Could you check a few things on this drawing? It's one solid part, dimensions in mm from its lowest x, y, z. Give positions to 0.01 mm unless a question says otherwise; leave off trailing zeros. Loops run counter-clockwise (first coordinate to the right, second up) from the corner with the lowest first, then second, coordinate; pieces in that order, holes last. Notation, with made-up numbers: (-23.5, -39.75) - (25.5, -39.75) arc R21 ccw to (25.5, -29.75) - close; hole circle Ø4 at (19, 67). An arc over 180 degrees is marked (long way). Use a Markdown table: item, result.
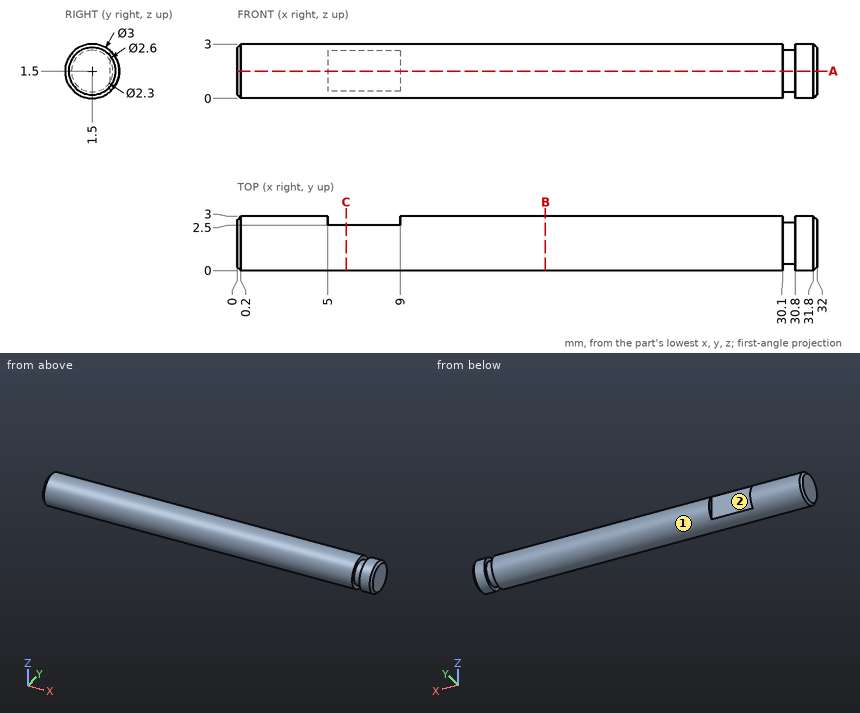
(1) Will this pin go through, and if not, where does the flat tip stop? pin 1 (0.7 mm diameter, centred on x = 6.5, z = 1.5, fed in from +Y).
A:
| item | result |
|---|---|
| pin 1 | y = 2.5 |
(2) Suppose I cut it at C-C on x = 6. Write out the boundary of the cut face in (y, z).
A:
| item | result |
|---|---|
| outline | (2.5, 0.38) - (2.5, 2.62) arc R1.5 ccw (long way) to start |
(3) Suppose I cut it at A-A on z = 1.5. Write out the boundary of the cut face in (x, y), plus the area to 3 significant figures.
A:
| item | result |
|---|---|
| outline | (0, 0.2) - (0.2, 0) - (30.1, 0) - (30.1, 0.35) - (30.8, 0.35) - (30.8, 0) - (31.8, 0) - (32, 0.2) - (32, 2.8) - (31.8, 3) - (30.8, 3) - (30.8, 2.65) - (30.1, 2.65) - (30.1, 3) - (9, 3) - (9, 2.5) - (5, 2.5) - (5, 3) - (0.2, 3) - (0, 2.8) - close |
| area | 93.4 mm2 |
(4) Suppose I cut it at B-B on x = 17. Write out the boundary of the cut face in (y, z).
A:
| item | result |
|---|---|
| outline | circle Ø3 at (1.5, 1.5) |
(5) We'd pull the mould along X, two halves only. Please class the marked faces 1 and 2: pulls with the +X half, pulls with the -X half, needs draft (parallel to the pull), parting line crosses it, or undercut.
A:
| item | result |
|---|---|
| face 1 | needs draft |
| face 2 | undercut |
(6) If I drill on line 1 (X direction, y = 2.8, z = 1.15); line 2 (X direction, y = 0.75, z = 0.45); line 3 (Z direction, x = 14.5, y = 0.5), over which ranges is the centre line in solid material (lowest first)?
A:
| item | result |
|---|---|
| line 1 | 0.05 to 5, 9 to 30.1, 30.8 to 31.95 |
| line 2 | 0 to 30.1, 30.8 to 32 |
| line 3 | 0.38 to 2.62 |
